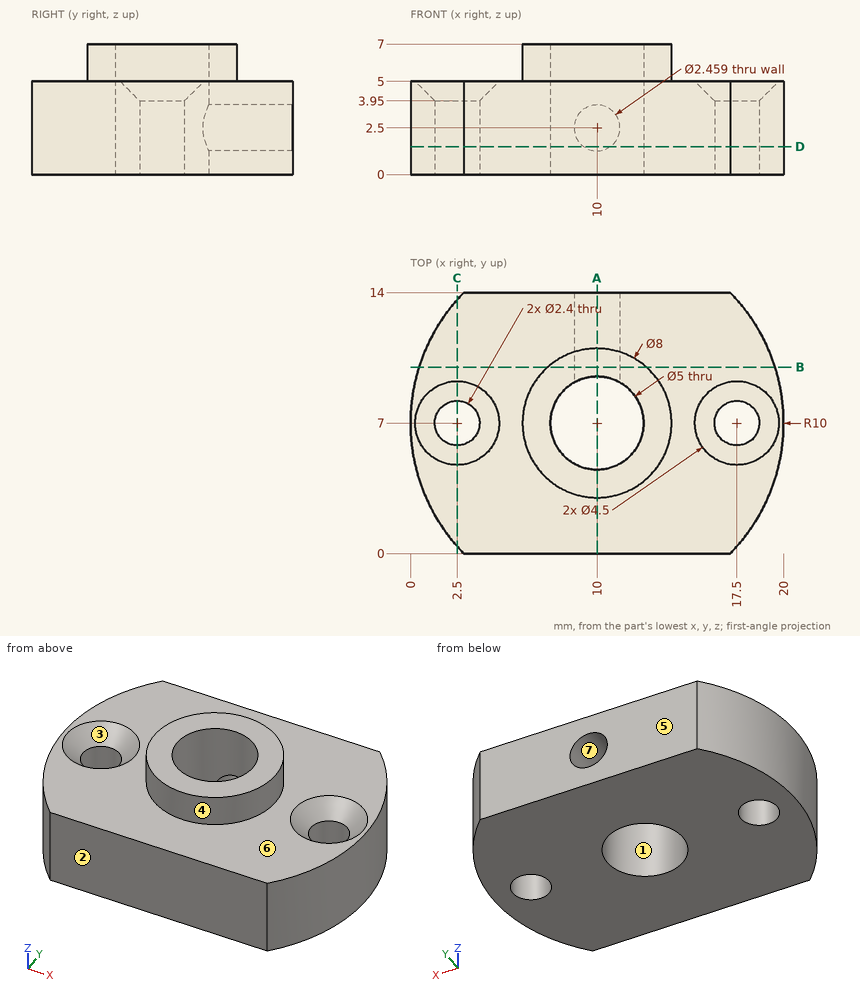
Geometry: see drawing. Coordinates: mm, zero at the bounding-box minimum. A direction names the side the tool comes from. Give positions to 0.01 mm unless a question says otherwise; leave off trailing zeros. Loops run counter-clockwise (first coordinate to the right, second up) from the corner with the lowest first, then second, coordinate; pieces in that order, holes last. Notation, with made-up numbers: (63, 78.5) - (69, 78.5) arc R23 cw to (69, 92.5) - close; hole circle Ø4 at (36, 84). An arc over 180 degrees is marked (long way). Use CSV: the item, a comma, the result in double quotes.
1) Cut plane B-B (y = 10). Output: boundary loops of the cut face in (x, z), and give its area (3 significant figures).
Worked out:
outline,"(0.46, 0) - (19.54, 0) - (19.54, 5) - (12.65, 5) - (12.65, 7) - (7.35, 7) - (7.35, 5) - (0.46, 5) - close; hole circle Ø2.46 at (10, 2.5)"
area,"101 mm^2"
2) Set-up query: the marked faces 5, 6 and 7. Return all of +Z, -Z, +X, -X, +Y, -Y with unobstructed straight access to the full face (end or side cutting, diameter ignored); none if empty.
Worked out:
face 5,"+Z, -Z, +X, -X, +Y"
face 6,"+Z"
face 7,"+Y"
3) Pin query (flat end, axial travel): P1, Ø1, axis at x = 4.5, y = 10, coming from the +Z side; P2, Ø3, axis at x = 10, y = 7, coming from the -Z side; P3, Ø3, axis at x = 17.5, y = 7, coming from the +Z side. Return the tip coordinate at first contact, or that it passes through.
Worked out:
P1,"stops at z = 5"
P2,"passes through"
P3,"stops at z = 4.25"
4) Line query: line 1 (X direction, y = 7, z = 3); line 2 (X direction, y = 7.75, z = 2.5) (3 decimals); line 3 (Z direction, x = 10, y = 10.1). Output: solid intervals per line, ascending.
Worked out:
line 1,"x = 0 to 1.3, 3.7 to 7.5, 12.5 to 16.3, 18.7 to 20"
line 2,"x = 0.028 to 1.563, 3.437 to 7.615, 12.385 to 16.563, 18.437 to 19.972"
line 3,"z = 0 to 1.27, 3.73 to 7"
5) Cut plane A-A (x = 10). Output: boundary loops of the cut face in (y, z).
Worked out:
outline,"(0, 0) - (4.5, 0) - (4.5, 7) - (3, 7) - (3, 5) - (0, 5) - close; (9.5, 0) - (14, 0) - (14, 1.27) - (9.5, 1.27) - close; (9.5, 3.73) - (14, 3.73) - (14, 5) - (11, 5) - (11, 7) - (9.5, 7) - close"
6) Mould query, pull axis X, two halves, no side actions, for the marked faces 1, 2, 3 and 4. Classes: +X half, -X half, draft (parallel to the pull), parting line (faces both ways), or undercut.
Worked out:
face 1,"undercut"
face 2,"draft"
face 3,"undercut"
face 4,"parting line"
7) Cut plane D-D (z = 1.5). Output: boundary loops of the cut face in (x, y), and give its area (3 significant figures).
Worked out:
outline,"(2.86, 0) - (17.14, 0) arc R10 ccw to (17.14, 14) - (10.72, 14) - (10.72, 9.4) arc R2.5 cw (long way) to (9.28, 9.4) - (9.28, 14) - (2.86, 14) arc R10 ccw to start; hole circle Ø2.4 at (2.5, 7); hole circle Ø2.4 at (17.5, 7)"
area,"220 mm^2"
8) Cut plane C-C (x = 2.5). Output: boundary loops of the cut face in (y, z), and give its area (3 significant figures).
Worked out:
outline,"(0.39, 0) - (5.8, 0) - (5.8, 3.95) - (4.75, 5) - (0.39, 5) - close; (8.2, 0) - (13.61, 0) - (13.61, 5) - (9.25, 5) - (8.2, 3.95) - close"
area,"53.0 mm^2"
